from build123d import *

# Parameters (mm, degrees)
EXTRUDE008_START = 76.7
SKETCH009_R      = 3.05
EXTRUDE008_DEPTH = 923.3
EXTRUDE007_START = -5
SKETCH008_W      = 25.1
SKETCH008_H      = 16
EXTRUDE007_DEPTH = 75
EXTRUDE006_DEPTH = 60
SKETCH004_R      = 2.325
EXTRUDE005_DEPTH = 150
EXTRUDE004_DEPTH = 2.2
EXTRUDE003_DEPTH = 50
EXTRUDE001_DEPTH = 107.5
SKETCH_W         = 69.2
SKETCH_H         = 215
EXTRUDE_DEPTH    = 30.2


with BuildPart() as extrude008:
    # Sketch009 → Extrude008 (new body)
    with BuildSketch(Plane.XZ.offset(EXTRUDE008_START)):
        with Locations((0, 4.7)):
            Circle(SKETCH009_R)
    extrude(amount=EXTRUDE008_DEPTH)


with BuildPart() as extrude007:
    # Sketch008 → Extrude007 (new body)
    with BuildSketch(Plane.XY.offset(EXTRUDE007_START)):
        with Locations((-15.05, 62.5)):
            Rectangle(SKETCH008_W, SKETCH008_H)
        with Locations((15.05, 62.5)):
            Rectangle(SKETCH008_W, SKETCH008_H)
        with Locations((-15.05, 31.5)):
            Rectangle(SKETCH008_W, SKETCH008_H)
        with Locations((15.05, 31.5)):
            Rectangle(SKETCH008_W, SKETCH008_H)
        with Locations((15.05, 10.5)):
            Rectangle(SKETCH008_W, SKETCH008_H)
        with Locations((-15.05, 10.5)):
            Rectangle(SKETCH008_W, SKETCH008_H)
    extrude(amount=-EXTRUDE007_DEPTH)


with BuildPart() as part_mirroring002:
    # Part__Mirroring002: instance of Extrude007
    add(extrude007.part.mirror(Plane(origin=(0, 0, 0), x_dir=(1, 0, 0), z_dir=(0, 1, 0))))


with BuildPart() as screwslotupper:
    # Sketch006 → Loft section 0
    with BuildSketch(Plane.XY):
        with BuildLine():
            ThreePointArc((-1.2, 48.75), (-3.6, 46.35), (-1.2, 43.95))
            Line((-1.2, 43.95), (1.2, 43.95))
            ThreePointArc((1.2, 43.95), (3.6, 46.35), (1.2, 48.75))
            Line((1.2, 48.75), (-1.2, 48.75))
        make_face()
    # Sketch007 → Loft section 1
    with BuildSketch(Plane.XY.offset(-30)):
        with BuildLine():
            ThreePointArc((-1.2, 48.75), (-3.6, 46.35), (-1.2, 43.95))
            Line((-1.2, 43.95), (18.520508, 43.95))
            ThreePointArc((18.520508, 43.95), (20.920508, 46.35), (18.520508, 48.75))
            Line((18.520508, 48.75), (-1.2, 48.75))
        make_face()
    loft()


with BuildPart() as screwslotlower:
    # Part__Mirroring001: instance of ScrewSlotUpper
    add(screwslotupper.part.mirror(Plane(origin=(0, 0, 0), x_dir=(1, 0, 0), z_dir=(0, 1, 0))))


with BuildPart() as anglefacecutout:
    # Sketch005 → Extrude006 (new body, symmetric)
    with BuildSketch(Plane.YZ):
        Polygon((-117.5, 9.68), (-117.5, 30.2), (72.5, 30.2), align=None)
    extrude(amount=EXTRUDE006_DEPTH, both=True)


with BuildPart() as securityhole:
    # Sketch004 → Extrude005 (new body)
    with BuildSketch(Plane.XZ):
        with Locations((0, 4.7)):
            Circle(SKETCH004_R)
    extrude(amount=EXTRUDE005_DEPTH)


with BuildPart() as mountingsquares:
    # Sketch001 → Extrude004 (new body)
    with BuildSketch(Plane.XY):
        Polygon((0, 51.2), (-8.3, 51.2), (-8.3, 46.35), (-8.3, 41.5), (0, 41.5), (8.3, 41.5), (8.3, 46.35), (8.3, 51.2), align=None)
        Polygon((0, -51.2), (8.3, -51.2), (8.3, -46.35), (8.3, -41.5), (0, -41.5), (-8.3, -41.5), (-8.3, -46.35), (-8.3, -51.2), align=None)
    extrude(amount=-EXTRUDE004_DEPTH)


with BuildPart() as topbottomanglecutout:
    # Sketch003 → Extrude003 (new body, symmetric)
    with BuildSketch(Plane.YZ):
        Polygon((-77.5, 30.2), (-95.132698, -69.8), (-145.132698, -69.8), (-145.132698, 30.2), (-95.132698, 30.2), align=None)
        Polygon((77.5, 30.2), (95.132698, -69.8), (145.132698, -69.8), (145.132698, 30.2), (95.132698, 30.2), align=None)
    extrude(amount=EXTRUDE003_DEPTH, both=True)


with BuildPart() as extrude001:
    # Sketch002 → Extrude001 (new body, symmetric)
    with BuildSketch(Plane.XZ):
        Polygon((0, 0), (-34.6, 0), (-34.6, 30.2), (-39.925075, 0), (48.975355, -51.326687), (34.6, 30.2), (34.6, 0), align=None)
    extrude(amount=EXTRUDE001_DEPTH, both=True)


with BuildPart() as cut001:
    # Sketch → Extrude (new body)
    with BuildSketch(Plane.XY):
        Rectangle(SKETCH_W, SKETCH_H)
        Polygon((29.6, 72.5), (-29.6, 72.5), (-29.6, -72.5), (0, -72.5), (29.6, -72.5), (29.6, 0), align=None, mode=Mode.SUBTRACT)
    extrude(amount=EXTRUDE_DEPTH)

    # Fusion: union Extrude001
    add(extrude001.part)

    # Cut: cut TopBottomAngleCutout
    add(topbottomanglecutout.part, mode=Mode.SUBTRACT)

    # Cut001: cut MountingSquares
    add(mountingsquares.part, mode=Mode.SUBTRACT)


with BuildPart() as cut008:
    # Part__Mirroring: instance of Cut001
    add(cut001.part.mirror(Plane(origin=(0, 0, 0), x_dir=(0, -1, 0), z_dir=(1, 0, 0))))

    # Cut002: cut SecurityHole
    add(securityhole.part, mode=Mode.SUBTRACT)

    # Cut003: cut AngleFaceCutout
    add(anglefacecutout.part, mode=Mode.SUBTRACT)

    # Cut004: cut ScrewSlotUpper
    add(screwslotupper.part, mode=Mode.SUBTRACT)

    # Cut005: cut ScrewSlotLower
    add(screwslotlower.part, mode=Mode.SUBTRACT)

    # Cut006: cut Part__Mirroring002
    add(part_mirroring002.part, mode=Mode.SUBTRACT)

    # Cut007: cut Extrude007
    add(extrude007.part, mode=Mode.SUBTRACT)

    # Cut008: cut Extrude008
    add(extrude008.part, mode=Mode.SUBTRACT)


solid = cut008.part
Build history of the part. All positions in model axes, mm. A direction names the side the tool comes from. Round coordinates to 2 decimals unless told otherwise and drop trailing zeros. Write each loop counter-clockwise with the first axis right and the second up, starting at its lowest first coordinate (ties: lowest second). Pieces come first, ordered by that corner, then holes. Notation, with made-up numbers: M 87.25,57.5 L 139.25,57.5 A16 ccw 139.25,79.5 Z; hole C 73.25,16.25 d10. An arc over 180 degrees is marked long. Answer as a JSON object with one key per item and string values. Group by question number.
(1) Cut at B-B (y = -7.5). Give the cut face in (x, z), and give its area (3 significant figures).
(2) Cut at A-A (z = 4.7). Give the cut face in (x, y) (3 decimals).
(3) Flat gauge pins, fed straight in: pin 1 (6 mm diameter, centred on x = 25, y = -45.5, fed in from -Z); pin 2 (17.5 mm diameter, centred on y = 61, z = -12.5, fed in from -X); pin 3 (2 mm diameter, centred on x = 7, y = 26, fed in from -Z). Where does each tip first touch, or does it go through?
(4) Mould opens along X. For faces 3 (the flat face through (-0.4, -72.5, 7.2)), 4 (the flat face through (-43.486, -1.286, -20.193)) say: pulls with the +X half, pulls with the -X half, needs draft (parallel to the pull), parting line crosses it, or undercut.
(5) Drill centre lines: L1, parallel to X at y = -81.2, z = 4.7; L2, parallel to X at y = 26, z = 20; L3, parallel to Y at x = 10, z = 6. Where is each one in solid material? Low to high.
(6) Which spindle directions (+Z, -Z, +X, -X, +Y, -Y) get a long thin tool onto all of the face, cutting with end or side? Do faces 1 (the flat face through (12, -18.5, -11)), 2 (the flat face through (29.6, 1, 12)). Say none if no direction does.
(7) Cut at D-D (z = -14.5). Give the number of separate pieces and of enclosed holes in the cut face, and give its area (3 significant figures).
(8) Cut at C-C (x = -42.5). Give the cut face in (y, z).
Responses:
{
 "1": {"outline": "M -48.98,-51.33 L -27.6,-38.99 L -27.6,-5 L -2.5,-5 L -2.5,-24.49 L 2.5,-21.61 L 2.5,-5 L 27.6,-5 L 27.6,-7.12 L 39.93,0 L 36.12,21.56 L 29.6,21.56 L 29.6,0 L -29.6,0 L -29.6,21.56 L -36.12,21.56 Z", "area": "1,510 mm2"},
 "2": {"outline": "M -39.096,-81.996 L -3.05,-81.996 L -3.05,-76.7 L -2.325,-76.7 L -2.325,-72.5 L -29.6,-72.5 L -29.6,72.5 L 29.6,72.5 L 29.6,-72.5 L 2.325,-72.5 L 2.325,-76.7 L 3.05,-76.7 L 3.05,-81.996 L 39.096,-81.996 L 39.096,81.996 L -39.096,81.996 Z"},
 "3": {"pin 1": "stops at z = -10.35", "pin 2": "stops at x = -43.67", "pin 3": "stops at z = -5"},
 "4": {"face 3": "undercut", "face 4": "pulls with the -X half"},
 "5": {"L1": "x = -39.1 to -3.05, 3.05 to 39.1", "L2": "x = -36.4 to -29.6, 29.6 to 36.4", "L3": "y = -81.77 to -72.5, 72.5 to 81.77"},
 "6": {"face 1": "-Z", "face 2": "+Z"},
 "7": {"separate pieces": "1", "enclosed holes": "8", "area": "6,050 mm2"},
 "8": {"outline": "M -91.22,-47.59 L 91.22,-47.59 L 85.4,-14.6 L -85.4,-14.6 Z"}
}
